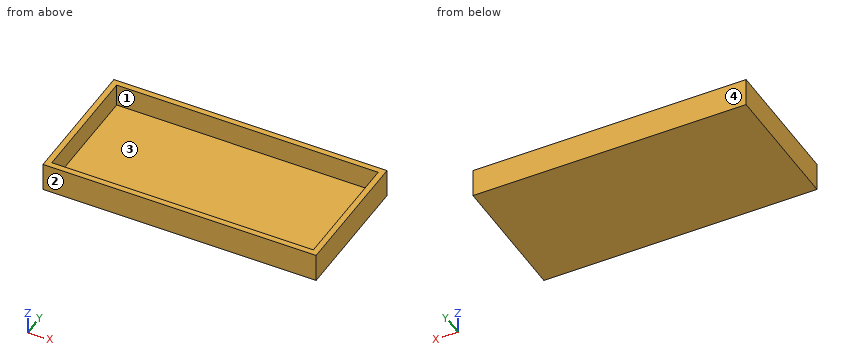
from build123d import *

# Parameters (mm, degrees)
F0_W     = 115.000024
F0_H     = 53.999892
F1_DEPTH = 10
F2_T     = 2.54


with BuildPart() as f1:
    # F0 (on Top) → F1 (new body)
    with BuildSketch(Plane.XY):
        with Locations((6.700012, 0.2917969662)):
            Rectangle(F0_W, F0_H)
    extrude(amount=F1_DEPTH)

    # F2
    f2_openings = [f1.faces().sort_by_distance(p)[0] for p in [
        (6.700012, 0.291797, 10),
    ]]
    offset(amount=F2_T, openings=f2_openings, kind=Kind.INTERSECTION)


solid = f1.part
Verification items for the finished model (mm, model axes). Face numbers are marked on the shaded views. A direction names the side the tool comes from. Give positions to 0.01 mm unless a question says otherwise; leave off trailing zeros. Write each loop counter-clockwise with the first axis right and the second up, starting at its lowest first coordinate (ties: lowest second). Pieces come first, ordered by that corner, then holes. Notation, with made-up numbers: M 67.25,9.5 L 85.25,9.5 A18 cw 85.25,13.5 Z; hole C -2.75,44.5 d8. An arc over 180 degrees is marked long. Use CSV: the item, a comma, the result in double quotes.
1) Material ranges on line 1 along X through (y, z) = (16, 3.5); line 2 along Y through (x, z) = (55, 5.5); line 3 along Z through (x, y) = (-16, 5), recorded low to high.
Final values:
line 1,"-53.34 to -50.8, 64.2 to 66.74"
line 2,"-29.25 to -26.71, 27.29 to 29.83"
line 3,"-2.54 to 0"
2) Access from +Z, -Z, +X, -X, +Y, -Y to the whole of each face (thin tool, end or side, straight path). Record for the marked faces 3 and 4.
Final values:
face 3,"+Z"
face 4,"+Z, -Z, +X, -X, +Y"
3) Cross-section at A-A (z = 7). Enter the section's corners in (x, y), plus the area to 3 significant figures.
Final values:
outline,"M -53.34,-29.25 L 66.74,-29.25 L 66.74,29.83 L -53.34,29.83 Z; hole M -50.8,-26.71 L 64.2,-26.71 L 64.2,27.29 L -50.8,27.29 Z"
area,"884 mm²"
4) Cross-section at B-B (x = 17.5). Enter the section's corners in (y, z).
Final values:
outline,"M -29.25,-2.54 L 29.83,-2.54 L 29.83,10 L 27.29,10 L 27.29,0 L -26.71,0 L -26.71,10 L -29.25,10 Z"
5) Release check for a two-part mould opening along X. For the marked faces 1 and 2 record: released by +X, released by -X, zero draft, split by the parting line, or undercut.
Final values:
face 1,"undercut"
face 2,"zero draft"
6) Cross-section at C-C (y = -10). Enter the section's corners in (x, z).
Final values:
outline,"M -53.34,-2.54 L 66.74,-2.54 L 66.74,10 L 64.2,10 L 64.2,0 L -50.8,0 L -50.8,10 L -53.34,10 Z"
